Part model, mm, in its own coordinate system. Face numbers are marked on the shaded views. A direction names the side the tool comes from. Round coordinates to 2 decimals unless told otherwise and drop trailing zeros. Loops run counter-clockwise (first coordinate to the right, second up) from the corner with the lowest first, then second, coordinate; pieces in that order, holes last. Notation, with made-up numbers: (-18.75, -30) -> (40.25, -30) arc R17 cw to (40.25, -6) -> close; hole circle Ø10 at (52, -37.75). An arc over 180 degrees is marked (long way). Answer as CSV lines item,"result".
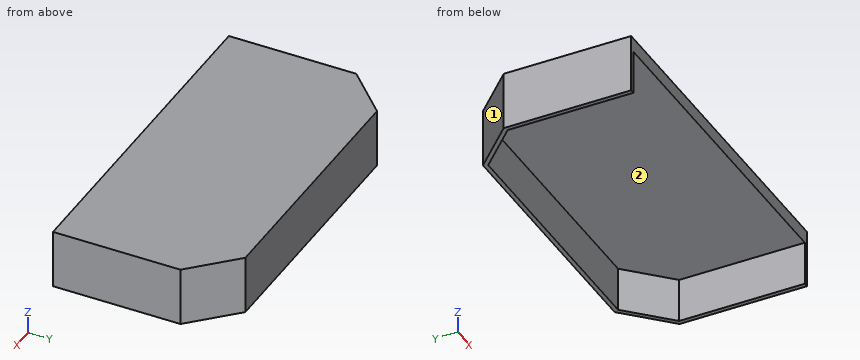
Solid Edge part; units mm, degrees
sketch "Sketch1" plane through (0, 0, 0) normal (0, 0, 1) x (1, 0, 0)
  line L0 (-115.5, -115.5) -> (115.5, -115.5)
  line L1 (115.5, -115.5) -> (115.5, 87.5)
  line L2 (115.5, 87.5) -> (87.5, 115.5)
  line L3 (87.5, 115.5) -> (-87.5, 115.5)
  line L4 (-87.5, 115.5) -> (-115.5, 87.5)
  line L5 (-115.5, 87.5) -> (-115.5, -115.5)
extrude "Protrusion1" add sketch "Sketch1" along normal blind 10
sketch "Sketch2" plane through (0, 0, 10) normal (0, 0, 1) x (1, 0, 0)
  line L0 (88.7426, 118.5) -> (-88.7426, 118.5)
  line L1 (-88.7426, 118.5) -> (-118.5, 88.7426)
  line L2 (-118.5, 88.7426) -> (-118.5, -118.5)
  line L3 (-118.5, -118.5) -> (118.5, -118.5)
  line L4 (118.5, -118.5) -> (118.5, 88.7426)
  line L5 (118.5, 88.7426) -> (88.7426, 118.5)
  line L6 (87.5, 115.5) -> (-87.5, 115.5)
  line L7 (-87.5, 115.5) -> (-115.5, 87.5)
  line L8 (-115.5, 87.5) -> (-115.5, -115.5)
  line L9 (-115.5, -115.5) -> (115.5, -115.5)
  line L10 (115.5, -115.5) -> (115.5, 87.5)
  line L11 (115.5, 87.5) -> (87.5, 115.5)
extrude "Protrusion2" add sketch "Sketch2" against normal blind 41
sketch "Sketch3" plane through (-118.5, -14.8787, -10.5) normal (-1, 0, 0) x (0, -1, 0)
  line L0 (103.6213, 20.5) -> (-14.9787, 20.5)
  line L1 (-14.9787, 20.5) -> (-14.9787, -20.5)
  line L2 (-14.9787, -20.5) -> (103.6213, -20.5)
  line L3 (103.6213, -20.5) -> (103.6213, 20.5)
extrude "Cutout1" cut sketch "Sketch3" against normal blind 280
Q1. Saw through at B-B, the plane z = -5.5. Write the cut outline in (x, y).
Geometry results:
outline,"(-118.5, 0.1) -> (-115.5, 0.1) -> (-115.5, 87.5) -> (-87.5, 115.5) -> (87.5, 115.5) -> (115.5, 87.5) -> (115.5, 0.1) -> (118.5, 0.1) -> (118.5, 88.74) -> (88.74, 118.5) -> (-88.74, 118.5) -> (-118.5, 88.74) -> close"
Q2. Saw through at A-A, the plane y = 19. Write the cut outline in (x, z), then the cut area to 3 significant figures.
Geometry results:
outline,"(-118.5, -31) -> (-115.5, -31) -> (-115.5, 0) -> (115.5, 0) -> (115.5, -31) -> (118.5, -31) -> (118.5, 10) -> (-118.5, 10) -> close"
area,"2,560 mm2"
Q3. Saw through at D-D, the plane y = 106. Write the cut outline in (x, z), then the cut area to 3 significant figures.
Geometry results:
outline,"(-101.24, -31) -> (-97, -31) -> (-97, 0) -> (97, 0) -> (97, -31) -> (101.24, -31) -> (101.24, 10) -> (-101.24, 10) -> close"
area,"2,290 mm2"
Q4. Which spindle directions (+Z, -Z, +X, -X, +Y, -Y) get a long thin tool onto all of the face, cutting with end or side? Do the marked faces 1 and 2. Say none if no direction does.
Geometry results:
face 1,"+Z, -Z, -X, +Y"
face 2,"-Z, -Y"
Q5. Saw through at C-C, the plane x = 8. Write the cut outline in (y, z), then the cut area to 3 significant figures.
Geometry results:
outline,"(0.1, 0) -> (115.5, 0) -> (115.5, -31) -> (118.5, -31) -> (118.5, 10) -> (0.1, 10) -> close"
area,"1,280 mm2"
Q6. Drop flat-ended pins along their axis: P1, Ø1, axis at x = 27.5, y = 24, coming from the -Z side; P2, Ø1, axis at x = 12.5, z = -7.5, coming from the -Y side. Give the stop position or say it passes through.
Geometry results:
P1,"z = 0"
P2,"y = 115.5"
Q7. Drill centre lines: line 1 along X through (y, z) = (56.5, -17.5); line 2 along Y through (x, z) = (-55, -1.5); line 3 along Z through (x, y) = (-50.5, 43). Where is each one in solid material? Low to high.
Geometry results:
line 1,"-118.5 to -115.5, 115.5 to 118.5"
line 2,"115.5 to 118.5"
line 3,"0 to 10"
